from build123d import *

# Parameters (mm, degrees)
SALIENTE_EXTRUIR1_DEPTH = 25
REDONDEO1_R             = 12
CROQUIS2_R              = 7.75
CORTAR_EXTRUIR1_DEPTH   = 10
CROQUIS3_R              = 2.8
CORTAR_EXTRUIR2_DEPTH   = 10
CROQUIS4_R              = 8.5
SALIENTE_EXTRUIR3_DEPTH = 1
CROQUIS5_R              = 1.25
CORTAR_EXTRUIR3_DEPTH   = 1
REDONDEO2_R             = 4
REDONDEO3_R             = 4
CROQUIS6_R              = 1.5
CORTAR_EXTRUIR4_DEPTH   = 10


with BuildPart() as part:
    # Croquis1 → Saliente-Extruir1 (new body)
    with BuildSketch(Plane(origin=(0, 0, 0), x_dir=(1, 0, 0), z_dir=(0, 1, 0))):
        Polygon((-25.5, -40), (-22, -40), (-22, 0), (22, 0), (22, -40), (25.5, -40), (25.5, 3.5), (-25.5, 3.5), align=None)
    extrude(amount=SALIENTE_EXTRUIR1_DEPTH)

    # Redondeo1
    redondeo1_edges = [part.edges().sort_by_distance(p)[0] for p in [
        (23.75, 0, 40),
        (-23.75, 0, 40),
        (23.75, 25, 40),
        (-23.75, 25, 40),
    ]]
    fillet(redondeo1_edges, radius=REDONDEO1_R)

    # Croquis2 → Cortar-Extruir1 (cut)
    with BuildSketch(Plane.ZY.offset(25.5)):
        with Locations((28, 12.5)):
            Circle(CROQUIS2_R)
    extrude(amount=-CORTAR_EXTRUIR1_DEPTH, mode=Mode.SUBTRACT)

    # Croquis3 → Cortar-Extruir2 (cut)
    with BuildSketch(Plane(origin=(25.5, 0, 0), x_dir=(0, 0, -1), z_dir=(1, 0, 0))):
        with Locations((-28, 12.5)):
            Circle(CROQUIS3_R)
    extrude(amount=-CORTAR_EXTRUIR2_DEPTH, mode=Mode.SUBTRACT)

    # Croquis4 → Saliente-Extruir3 (add)
    with BuildSketch(Plane(origin=(25.5, 0, 0), x_dir=(0, 0, -1), z_dir=(1, 0, 0))):
        with Locations((-28, 12.5)):
            Circle(CROQUIS4_R)
    extrude(amount=SALIENTE_EXTRUIR3_DEPTH)

    # Croquis5 → Cortar-Extruir3 (cut)
    with BuildSketch(Plane(origin=(26.5, 0, 0), x_dir=(0, 0, -1), z_dir=(1, 0, 0))):
        with Locations((-28, 12.5)):
            Circle(CROQUIS5_R)
    extrude(amount=-CORTAR_EXTRUIR3_DEPTH, mode=Mode.SUBTRACT)

    # Redondeo2
    redondeo2_edges = [part.edges().sort_by_distance(p)[0] for p in [
        (22, 12.5, 0),
        (-22, 12.5, 0),
    ]]
    fillet(redondeo2_edges, radius=REDONDEO2_R)

    # Redondeo3
    redondeo3_edges = [part.edges().sort_by_distance(p)[0] for p in [
        (-25.5, 12.5, -3.5),
        (25.5, 12.5, -3.5),
    ]]
    fillet(redondeo3_edges, radius=REDONDEO3_R)

    # Croquis6 → Cortar-Extruir4 (cut)
    with BuildSketch(Plane(origin=(0, 0, -3.5), x_dir=(-1, 0, 0), z_dir=(0, 0, -1))):
        with Locations((-10, 12.5)):
            Circle(CROQUIS6_R)
        with Locations((10, 12.5)):
            Circle(CROQUIS6_R)
    extrude(amount=-CORTAR_EXTRUIR4_DEPTH, mode=Mode.SUBTRACT)


solid = part.part
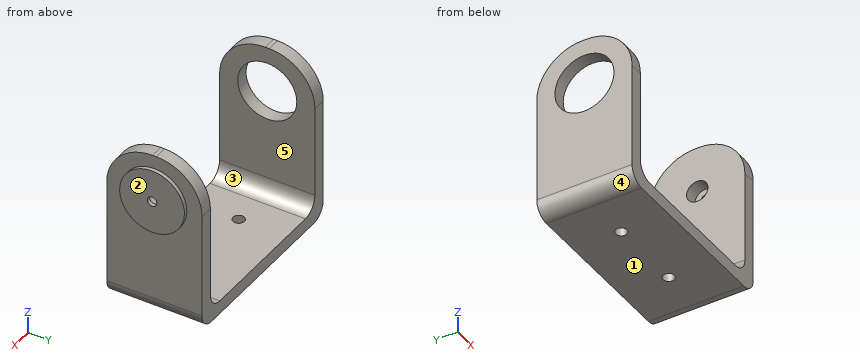
Verification items for the finished model (mm, model axes). Face numbers are marked on the shaded views. A direction names the side the tool comes from. Coordinates: 2 decimals unless noted, no trailing zeros. Write each loop counter-clockwise with the first axis right and the second up, starting at its lowest first coordinate (ties: lowest second). Pieces come first, ordered by that corner, then holes. Notation, with made-up numbers: (-4, 2.25) -> (23, 2.25) arc R15 ccw to (23, 14.25) -> close; hole circle Ø5 at (-17.5, 6.5). An arc over 180 degrees is marked (long way). One line per item, written item: value. Start each with the question number.
Q1. Access from +Z, -Z, +X, -X, +Y, -Y to the whole of each face (thin tool, end or side, straight path). Record for the marked faces 4 and 5.
Q2. Thickness scan on L1, parallel to X at y = 11, z = 19; L2, parallel to Y at x = 24, z = 28; L3, parallel to X at y = 4.25, z = 27. Record the ranges inside material, lowest first. Write a range as from..to.
Q3. Cross-section at B-B on x = 10. Enter the section's corners in (y, z).
Q4. Cross-section at C-C on y = 19. Enter the section's corners in (x, z).
Q5. Mould release check, pull along X, two halves, no side actions. Record for the marked faces 1, 2 and 3: pulls with the +X half, pulls with the -X half, needs draft (parallel to the pull), parting line crosses it, or undercut.
Q6. Cross-section at A-A on z = 6. Enter the section's corners in (x, y).
Q7. Cross-section at D-D on z = 23. Enter the section's corners in (x, y), and give its area (3 significant figures).
Q8. Go/stop test with flat-tipped pins: P1, Ø5, axis at y = 12.5, z = 28, coming from the -X side; P2, Ø14, axis at y = 12.5, z = 28, coming from the -X side; P3, Ø3, axis at x = 7.5, y = 22, coming from the +Z side. Record where each tip stops, or that it passes through.
Checked values:
1. face 4: -Z, -X, +Y, -Y
1. face 5: +Z, +Y, -Y
2. L1: x = -25.5..-22, 22..25.5
2. L2: y = 0..9.7, 15.3..25
2. L3: x = -25.5..-22, 22..26.5
3. outline: (0, -3.5) -> (11, -3.5) -> (11, 0) -> (0, 0) -> close; (14, -3.5) -> (25, -3.5) -> (25, 0) -> (14, 0) -> close
4. outline: (-25.5, 0.5) arc R4 ccw to (-21.5, -3.5) -> (21.5, -3.5) arc R4 ccw to (25.5, 0.5) -> (25.5, 22.52) -> (26.5, 22.52) -> (26.5, 33.48) -> (25.5, 33.48) -> (25.5, 38.39) -> (22, 38.39) -> (22, 4) arc R4 cw to (18, 0) -> (-18, 0) arc R4 cw to (-22, 4) -> (-22, 23.78) -> (-25.5, 23.78) -> close; (-25.5, 32.22) -> (-22, 32.22) -> (-22, 38.39) -> (-25.5, 38.39) -> close
5. face 1: needs draft
5. face 2: pulls with the +X half
5. face 3: undercut
6. outline: (-25.5, 0) -> (-22, 0) -> (-22, 25) -> (-25.5, 25) -> close; (22, 0) -> (25.5, 0) -> (25.5, 25) -> (22, 25) -> close
7. outline: (-25.5, 0) -> (-22, 0) -> (-22, 6.58) -> (-25.5, 6.58) -> close; (-25.5, 18.42) -> (-22, 18.42) -> (-22, 25) -> (-25.5, 25) -> close; (22, 0) -> (25.5, 0) -> (25.5, 5.63) -> (26.5, 5.63) -> (26.5, 19.37) -> (25.5, 19.37) -> (25.5, 25) -> (22, 25) -> close
7. area: 147 mm²
8. P1: stops at x = 25.5
8. P2: stops at x = 22
8. P3: stops at z = 0
